Work out the finished part from the listing and answer in its coordinate system (mm). Coordinates: 2 decimals unless noted, no trailing zeros. Order: outer loops, then holes, each group sorted by start corner. A loop starts at its lowest first (then second) coordinate and runs counter-clockwise, first axis right, second up. Notation, with made-up numbers: M -7.5,53 L 13.5,53 A18 ccw 13.5,58 Z; hole C -38,0 d11. An arc over 180 degrees is marked long. Answer in a Markdown table with one row per item. Add a question column.
Item 1: Consider line 1 (Y direction, x = 19, z = 16.25); line 2 (X direction, y = 137.5, z = 4); line 3 (X direction, y = 149, z = 16.75). Determine where each line is inside the solid, lowest interval first. Write a range as from..to.
Item 2: The part is cut by section C-C (z = 10). State how many separate pieces and enclosed holes the cut face has, then the cut area to 3 significant figures.
Item 3: Flat-ended cylindrical pins translate along their axes: pin 1 Ø12 at (y, z) = (10, 17) entering from +X; pin 2 Ø7.5 at (x, z) = (-91.5, 17.5) entering from +Y; pin 3 Ø7.5 at (y, z) = (137, 17) entering from -X. Find the tip coordinate at first contact, or state that the pin passes through.
Item 4: The part is cut by section B-B (x = -104.5). Write down the section's boundary in (y, z).
Item 5: The part is cut by section D-D (y = 118). Write down the section's boundary in (x, z).
Item 6: The part is cut by section A-A (y = 197). Write down the section's boundary in (x, z), then the cut area to 3 significant figures.
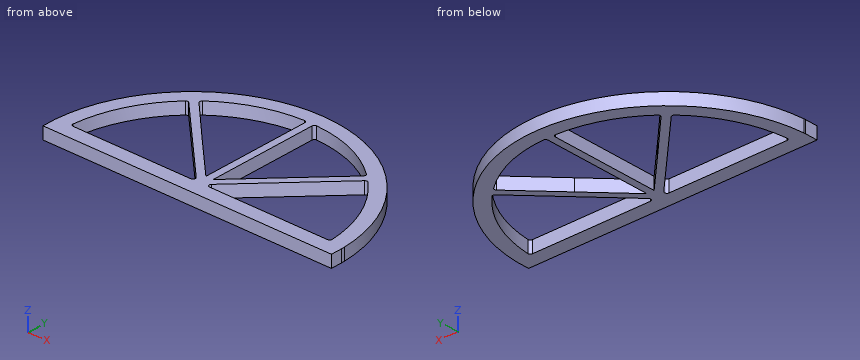
from build123d import *

# Parameters (mm, degrees)
F1_DEPTH = 25
F2_R     = 5
F3_R     = 5


with BuildPart() as f1:
    # F0 (on Top) → F1 (new body)
    with BuildSketch(Plane.XY):
        with BuildLine():
            Line((-299.905914, -16.159892), (-299.905914, -42.432796))
            Line((-299.905914, -42.432796), (300.094086, -42.432796))
            Line((300.094086, -42.432796), (300.094086, -18.9935))
            ThreePointArc((300.094086, -18.9935), (299.947953, -15.712251), (299.765939, -12.432796))
            ThreePointArc((299.765939, -12.432796), (0.032047, 269.577673), (-299.701846, -12.432796))
            ThreePointArc((-299.701846, -12.432796), (-299.809671, -14.296027), (-299.905914, -16.159892))
        make_face()
        with BuildLine():
            Line((-7.5, -12.432796), (-269.905914, -12.432796))
            ThreePointArc((-269.905914, -12.432796), (-245.019334, 84.882969), (-186.345143, 166.412347))
            Line((-186.345143, 166.412347), (-7.5, -12.432796))
        make_face(mode=Mode.SUBTRACT)
        with BuildLine():
            ThreePointArc((186.436841, 166.504045), (245.179328, 84.94326), (270.094086, -12.432796))
            Line((270.094086, -12.432796), (7.5, -12.432796))
            Line((7.5, -12.432796), (186.436841, 166.504045))
        make_face(mode=Mode.SUBTRACT)
        with BuildLine():
            Line((-7.5, 240.801209), (-7.5, 49.689975))
            Line((-7.5, 49.689975), (-7.5, 8.780407))
            Line((-7.5, 8.780407), (-86.31597, 87.596377))
            Line((-86.31597, 87.596377), (-174.624587, 176.925959))
            ThreePointArc((-174.624587, 176.925959), (-96.495237, 223.078456), (-7.5, 240.801209))
        make_face(mode=Mode.SUBTRACT)
        with BuildLine():
            Line((7.5, 8.780407), (7.5, 49.689975))
            Line((7.5, 49.689975), (7.5, 240.801209))
            ThreePointArc((7.5, 240.801209), (97.204461, 223.874551), (175.263477, 176.543885))
            Line((175.263477, 176.543885), (86.361819, 87.642226))
            Line((86.361819, 87.642226), (7.5, 8.780407))
        make_face(mode=Mode.SUBTRACT)
    extrude(amount=F1_DEPTH)

    # F2
    f2_edges = [f1.edges().sort_by_distance(p)[0] for p in [
        (-7.5, 240.801209, 12.5),
        (175.263477, 176.543885, 12.5),
        (270.094086, -12.432796, 12.5),
        (7.5, 240.801209, 12.5),
        (-186.345143, 166.412347, 12.5),
        (-269.905914, -12.432796, 12.5),
        (186.436841, 166.504045, 12.5),
        (-174.624587, 176.925959, 12.5),
    ]]
    fillet(f2_edges, radius=F2_R)

    # F3
    f3_edges = [f1.edges().sort_by_distance(p)[0] for p in [
        (7.5, -12.432796, 12.5),
        (-7.5, -12.432796, 12.5),
    ]]
    fillet(f3_edges, radius=F3_R)


solid = f1.part
Reply:
| question | item | result |
|---|---|---|
| 1 | line 1 | y = -42.43..-12.4, -0.93..20.28, 240.46..268.98 |
| 1 | line 2 | x = -248.72..-212.65, -157.43..-135.65, -7.5..7.5, 136.22..157.43, 212.84..248.79 |
| 1 | line 3 | x = -240.55..-203.09, -168.93..-147.02, -7.5..7.5, 147.72..168.93, 203.28..240.61 |
| 2 | separate pieces | 1 |
| 2 | enclosed holes | 4 |
| 2 | area | 54,200 mm2 |
| 3 | pin 1 | stops at x = 298.31 |
| 3 | pin 2 | stops at y = 256.46 |
| 3 | pin 3 | stops at x = -251.54 |
| 4 | outline | M -42.43,0 L -12.43,0 L -12.43,25 L -42.43,25 Z; M 84.57,0 L 105.99,0 L 105.99,25 L 84.57,25 Z; M 219.87,0 L 250.8,0 L 250.8,25 L 219.87,25 Z |
| 5 | outline | M -260.85,0 L -226.62,0 L -226.62,25 L -260.85,25 Z; M -137.93,0 L -116.37,0 L -116.37,25 L -137.93,25 Z; M -7.5,0 L 7.5,0 L 7.5,25 L -7.5,25 Z; M 116.72,0 L 137.93,0 L 137.93,25 L 116.72,25 Z; M 226.81,0 L 260.91,0 L 260.91,25 L 226.81,25 Z |
| 6 | outline | M -195.73,0 L -147.66,0 L -147.66,25 L -195.73,25 Z; M -7.5,0 L 7.5,0 L 7.5,25 L -7.5,25 Z; M 148.85,0 L 195.79,0 L 195.79,25 L 148.85,25 Z |
| 6 | area | 2,750 mm2 |
